Could you check a few things on this drawing? It's one solid part, dimensions in mm from its lowest x, y, z. A direction names the side the tool comes from. Give positions to 0.01 mm unless a question says otherwise; leave off trailing zeros. Order: outer loops, then holes, each group sorted by start corner. A loop starts at its lowest first (then second) coordinate and runs counter-clockwise, first axis right, second up. Notation, with made-up numbers: (59.25, 44) - (102.25, 44) arc R22 ccw to (102.25, 60) - close; hole circle Ø2 at (59.5, 13). An arc over 180 degrees is marked (long way). One line per question, with ' | ' between items. Start each with the question number.
1. For P1, Ø4.5, axis at y = 13, z = 30, coming from the +X side; P2, Ø4, axis at x = 116.5, z = 24, coming from the -Y side; P3, Ø4.5, axis at y = 8.5, z = 26, coming from the -X side; P4, Ø1.5, axis at x = 56.5, y = 5, coming from the -Z side (1 decimal), each with a flat end and sliding along its axis, tell me the tip position at first contact or that it passes through.
2. Imagine slicing it at C-C (z = 15.5). Please give me the cut outline in (x, y).
3. Imagine slicing it at D-D (y = 13.5). Please give me the cut outline in (x, z) (1 decimal).
4. Imagine slicing it at A-A (z = 25.5). Please give me the cut outline in (x, y).
5. I need wall thicknesses on probe 1 along X at (y, z) = (0.4, 25.5); probe 2 along Z at (x, y) = (153.7, 0.75); probe 3 along Z at (x, y) = (46, 15.5) (1 decimal). Which ranges of each line are inside material? Lowest first, please. Write a range as from..to.
6. Which directions (+Z, -Z, +X, -X, +Y, -Y) give clear straight access to the entire face, cutting with the end or side of a thin tool? Please do the marked faces 1, 2 and 3.
7. Imagine slicing it at B-B (x = 79). Please give me the cut outline in (y, z).
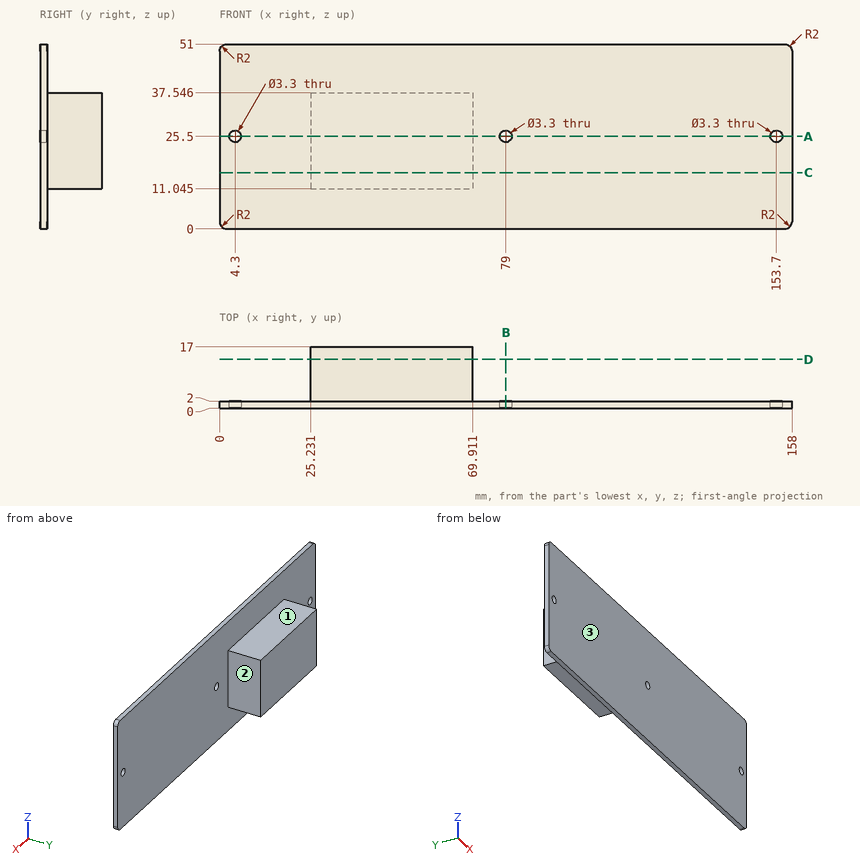
Results found:
1) P1: stops at x = 69.91 | P2: stops at y = 0 | P3: stops at x = 25.23 | P4: stops at z = 11
2) outline: (0, 0) - (158, 0) - (158, 2) - (69.91, 2) - (69.91, 17) - (25.23, 17) - (25.23, 2) - (0, 2) - close
3) outline: (25.2, 11) - (69.9, 11) - (69.9, 37.5) - (25.2, 37.5) - close
4) outline: (0, 0) - (2.65, 0) - (2.65, 2) - (0, 2) - close; (5.95, 0) - (77.35, 0) - (77.35, 2) - (69.91, 2) - (69.91, 17) - (25.23, 17) - (25.23, 2) - (5.95, 2) - close; (80.65, 0) - (152.05, 0) - (152.05, 2) - (80.65, 2) - close; (155.35, 0) - (158, 0) - (158, 2) - (155.35, 2) - close
5) probe 1: x = 0..2.65, 5.95..77.35, 80.65..152.05, 155.35..158 | probe 2: z = 0..23.85, 27.15..51 | probe 3: z = 11..37.5
6) face 1: +Z, +X, -X, +Y | face 2: +Z, -Z, +X, +Y | face 3: +Z, -Z, +X, -X, -Y
7) outline: (0, 0) - (2, 0) - (2, 23.85) - (0, 23.85) - close; (0, 27.15) - (2, 27.15) - (2, 51) - (0, 51) - close
